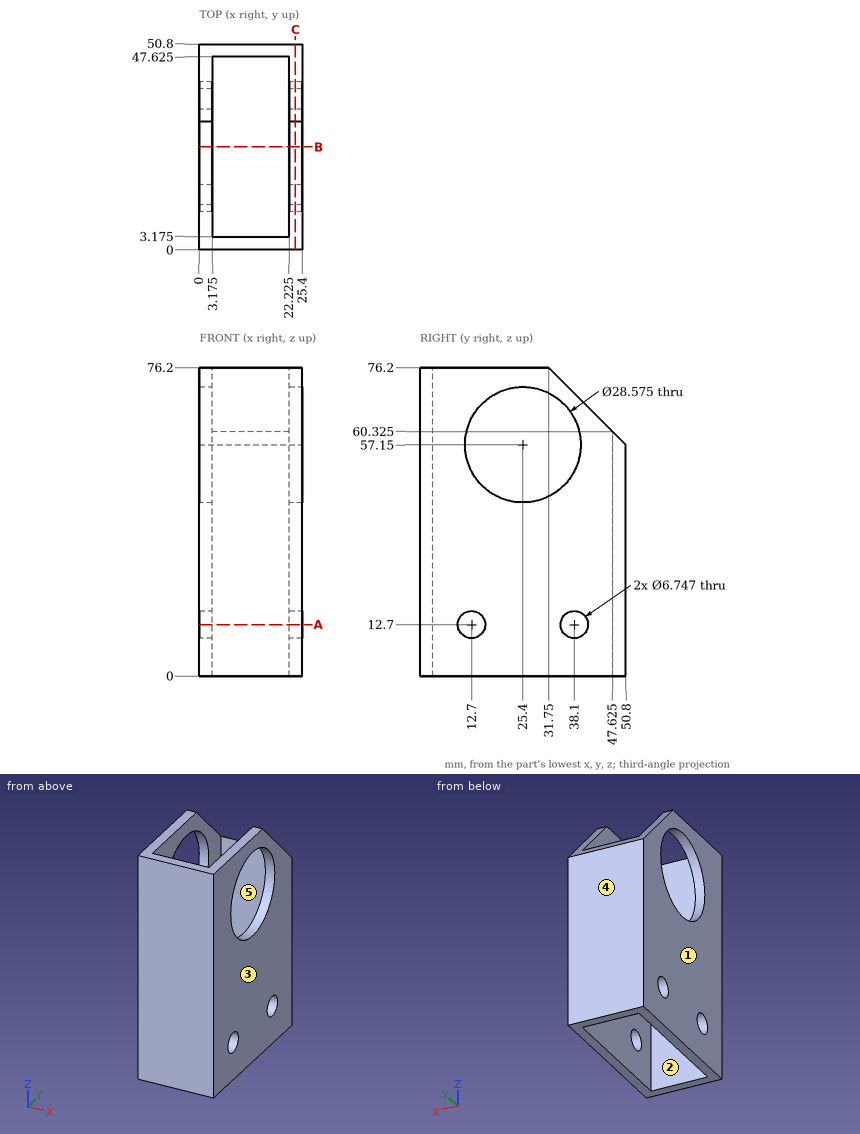
Print and shaded views of the part. All mm, measured from the part's lowest x, y and z. A direction names the side the tool comes from. Coordinates: 2 decimals unless noted, no trailing zeros. Order: outer loops, then holes, each group sorted by start corner. A loop starts at its lowest first (then second) coordinate and runs counter-clockwise, first axis right, second up.
(1) Tool access for the marked faces 1 and 2: list every direction of +Z, -Z, +X, -X, +Y, -Y with a clear straight run to the whole face (end or side of a thin tool).
Check sheet entries:
face 1: +Z, -Z, -X, +Y, -Y
face 2: +Z, -Z
(2) Slice it at C-C, the plane x = 23.75. State how many separate pieces and enclosed holes the cut face has, and give its area (3 significant figures).
Check sheet entries:
separate pieces: 1
enclosed holes: 3
area: 2,980 mm2
(3) Slice it at B-B, the plane y = 25.4. Write the cut outline in (x, z) (1 decimal).
Check sheet entries:
outline: (0, 0) - (3.2, 0) - (3.2, 42.9) - (0, 42.9) - close; (0, 71.4) - (3.2, 71.4) - (3.2, 76.2) - (0, 76.2) - close; (22.2, 0) - (25.4, 0) - (25.4, 42.9) - (22.2, 42.9) - close; (22.2, 71.4) - (25.4, 71.4) - (25.4, 76.2) - (22.2, 76.2) - close
(4) Pull direction Y, two halves, no side cores. Call the marked faces 3, 4 and 5: pulls with the +Y half, pulls with the -Y half, needs draft (parallel to the pull), parting line crosses it, or undercut.
Check sheet entries:
face 3: needs draft
face 4: pulls with the +Y half
face 5: undercut
(5) Slice it at A-A, the plane z = 12.7. Write the cut outline in (x, y) (1 decimal).
Check sheet entries:
outline: (0, 0) - (25.4, 0) - (25.4, 9.3) - (22.2, 9.3) - (22.2, 3.2) - (3.2, 3.2) - (3.2, 9.3) - (0, 9.3) - close; (0, 16.1) - (3.2, 16.1) - (3.2, 34.7) - (0, 34.7) - close; (0, 41.5) - (3.2, 41.5) - (3.2, 47.6) - (22.2, 47.6) - (22.2, 41.5) - (25.4, 41.5) - (25.4, 50.8) - (0, 50.8) - close; (22.2, 16.1) - (25.4, 16.1) - (25.4, 34.7) - (22.2, 34.7) - close
(6) Probe L1, parallel to Y at x = 1.7, z = 12.7; L2, parallel to X at y = 13, z = 41 (3 decimals); L3, parallel to Y at x = 14.5, z = 48 (3 decimals). List the from-to ranges inside material, lowest first.
Check sheet entries:
L1: y = 0 to 9.33, 16.07 to 34.73, 41.47 to 50.8
L2: x = 0 to 3.175, 22.225 to 25.4
L3: y = 0 to 3.175, 47.625 to 50.8
